Build history of the part. All positions in model axes, mm. A direction names the side the tool comes from. Coordinates: 2 decimals unless noted, no trailing zeros. Order: outer loops, then holes, each group sorted by start corner. A loop starts at its lowest first (then second) coordinate and runs counter-clockwise, first axis right, second up. Notation, with made-up numbers: (10.25, -7) - (16.25, -7) arc R21 ccw to (16.25, 7) - close; hole circle Ø10 at (22, 80). An arc over 180 degrees is marked (long way). Write each question's results on one line, items separated by ' | '. Start each with the question number.
Autodesk Inventor part; units mm, degrees
ref_plane "YZ Plane" through (0, 0, 0) normal (1, 0, 0) x (0, 1, 0)
ref_plane "XZ Plane" through (0, 0, 0) normal (0, 1, 0) x (-1, 0, 0)
ref_plane "XY Plane" through (0, 0, 0) normal (0, 0, 1) x (1, 0, 0)
sketch "スケッチ1" plane through (0, 0, 0) normal (0, 0, 1) x (1, 0, 0)
  line L0 (-47, 28.25) -> (-37.7144, 28.25)
  line L1 (47, 28.25) -> (47, 23.75)
  line L2 (47, -28.25) -> (-47, -28.25)
  line L3 (-47, -28.25) -> (-47, -11.5167)
  line L4 (-47, 28.25) -> (47, -28.25) construction
  line L5 (47, 28.25) -> (-47, -28.25) construction
  line L6 (0, 28.25) -> (0, -28.25) construction
  line L7 (-33, 9.4167) -> (-28, 9.4167) construction
  line L8 (-28, 9.4167) -> (-28, -9.4167) construction
  line L9 (-28, -9.4167) -> (-33, -9.4167) construction
  line L10 (-33, -9.4167) -> (-33, 9.4167) construction
  line L11 (-33, 9.4167) -> (-28, -9.4167) construction
  line L12 (-28, 9.4167) -> (-33, -9.4167) construction
  line L13 (-33.05, 9.4667) -> (-27.95, 9.4667)
  line L14 (-27.95, 9.4667) -> (-27.95, 7.3667) construction
  line L15 (-27.95, -9.4667) -> (-33.05, -9.4667)
  line L16 (-33.05, -9.4667) -> (-33.05, -7.3667) construction
  line L17 (-33.05, 9.4667) -> (-27.95, -9.4667) construction
  line L18 (-27.95, 9.4667) -> (-33.05, -9.4667) construction
  arc A0 (-33.05, 9.4667) -> (-33.05, 7.3667) centre (-33.05, 8.4167) ccw
  line L19 (-30.5, 9.4667) -> (-30.5, -9.4667) construction
  arc A1 (-27.95, 7.3667) -> (-27.95, 9.4667) centre (-27.95, 8.4167) ccw
  line L20 (-33.05, 7.3667) -> (-33.05, 9.4667) construction
  line L21 (-27.95, 7.3667) -> (-27.95, -7.3667)
  line L22 (-33.05, -7.3667) -> (-33.05, 7.3667)
  line L23 (-27.95, -7.3667) -> (-27.95, -9.4667) construction
  line L24 (33, 9.4167) -> (28, 9.4167) construction
  line L25 (28, 9.4167) -> (28, -9.4167) construction
  line L26 (28, -9.4167) -> (33, -9.4167) construction
  line L27 (33, -9.4167) -> (33, 9.4167) construction
  line L28 (33, 9.4167) -> (28, -9.4167) construction
  line L29 (28, 9.4167) -> (33, -9.4167) construction
  line L30 (33.05, 9.4667) -> (27.95, 9.4667)
  line L31 (27.95, 9.4667) -> (27.95, 7.3667) construction
  line L32 (27.95, -9.4667) -> (33.05, -9.4667)
  line L33 (33.05, -9.4667) -> (33.05, -7.3667) construction
  line L34 (33.05, 9.4667) -> (27.95, -9.4667) construction
  line L35 (27.95, 9.4667) -> (33.05, -9.4667) construction
  arc A2 (33.05, 7.3667) -> (33.05, 9.4667) centre (33.05, 8.4167) ccw
  line L36 (30.5, 9.4667) -> (30.5, -9.4667) construction
  arc A3 (27.95, 9.4667) -> (27.95, 7.3667) centre (27.95, 8.4167) ccw
  line L37 (33.05, 7.3667) -> (33.05, 9.4667) construction
  line L38 (27.95, 7.3667) -> (27.95, -7.3667)
  line L39 (33.05, -7.3667) -> (33.05, 7.3667)
  line L40 (27.95, -7.3667) -> (27.95, -9.4667) construction
  line L41 (-52, 9.4167) -> (-52, -9.4167)
  line L42 (-52, 9.4167) -> (-47, 9.4167)
  arc A4 (-47, 9.4167) -> (-47, 11.5167) centre (-47, 10.4667) ccw
  line L43 (-47, 11.5167) -> (-47, 23.75)
  line L44 (-47, -11.5167) -> (-47, 11.5167)
  line L45 (52, 9.4167) -> (52, -9.4167)
  line L46 (52, 9.4167) -> (47, 9.4167)
  arc A5 (47, 11.5167) -> (47, 9.4167) centre (47, 10.4667) ccw
  line L47 (47, 11.5167) -> (47, -11.5167)
  line L48 (47, -11.5167) -> (47, -28.25)
  line L49 (-52, 0) -> (52, 0) construction
  line L50 (-52, -9.4167) -> (-47, -9.4167)
  arc A6 (-47, -11.5167) -> (-47, -9.4167) centre (-47, -10.4667) ccw
  arc A7 (47, -9.4167) -> (47, -11.5167) centre (47, -10.4667) ccw
  line L51 (52, -9.4167) -> (47, -9.4167)
  line L52 (-33.05, 0) -> (-27.95, 0) construction
  arc A8 (-33.05, -7.3667) -> (-33.05, -9.4667) centre (-33.05, -8.4167) ccw
  arc A9 (-27.95, -9.4667) -> (-27.95, -7.3667) centre (-27.95, -8.4167) ccw
  arc A10 (27.95, -7.3667) -> (27.95, -9.4667) centre (27.95, -8.4167) ccw
  arc A11 (33.05, -9.4667) -> (33.05, -7.3667) centre (33.05, -8.4167) ccw
  arc A12 (-47, 24.0838) -> (-37.7144, 28.25) centre (-44.75, 31.5) ccw
  arc A13 (37.7144, 28.25) -> (47, 24.0838) centre (44.75, 31.5) ccw
  line L53 (-47, 24.0838) -> (-47, 28.25)
  line L54 (-37.7144, 28.25) -> (47, 28.25)
  arc A14 (-37.7144, 28.25) -> (-47, 24.0838) centre (-44.75, 31.5) ccw
  arc A15 (47, 24.0838) -> (37.7144, 28.25) centre (44.75, 31.5) ccw
  line L55 (-44.75, 23.75) -> (-47, 23.75)
  line L56 (44.75, 23.75) -> (47, 23.75)
  line L57 (-47, 23.75) -> (-47, 24.0838)
  line L58 (47, 23.75) -> (47, 11.5167)
  line L59 (-23, 23.25) -> (23, 23.25)
  line L60 (23, 23.25) -> (23, -23.25)
  line L61 (23, -23.25) -> (-23, -23.25)
  line L62 (-23, -23.25) -> (-23, 23.25)
  line L63 (-23, 23.25) -> (23, -23.25) construction
  line L64 (23, 23.25) -> (-23, -23.25) construction
  line L65 (-42, 8.25) -> (42, 8.25) construction
  line L66 (42, 8.25) -> (42, -18.25) construction
  line L67 (42, -18.25) -> (-42, -18.25) construction
  line L68 (-42, -18.25) -> (-42, 8.25) construction
  line L69 (-42, 8.25) -> (42, -18.25) construction
  line L70 (42, 8.25) -> (-42, -18.25) construction
  circle A16 centre (-39, 5.25) radius 1.25
  line L71 (-42, -5) -> (42, -5) construction
  circle A17 centre (-39, -15.25) radius 1.25
  circle A18 centre (39, 5.25) radius 1.25
  circle A19 centre (39, -15.25) radius 1.25
  point P0 (0, 0)
  point P1 (-30.5, 0)
  point P2 (30.5, 0)
  point P3 (0, 0)
  point P4 (-30.5, 0)
  point P5 (-30.5, 0)
  point P6 (0, 0)
  point P7 (0, 0)
  point P8 (47, 9.4167)
  point P9 (47, 9.4167)
  point P10 (0, -5)
  point P11 (0, -5)
  dimension "d0" = 94
  dimension "d1" = 56.5
  dimension "d2" = 5
  dimension "d3" = 18.8333
  dimension "d4" = 1.05
  dimension "d5" = 0.05
  dimension "d6" = 0.05
  dimension "d7" = 56
  dimension "d10" = 1.05
  dimension "d11" = 5
  dimension "d34" = 18.8333
  dimension "d40" = 31.5
  dimension "d41" = 89.5
  dimension "d42" = 15.5
  dimension "d43" = 52
  dimension "d60" = 5
  dimension "d63" = 5
  dimension "d69" = 5
  dimension "d70" = 20
  dimension "d71" = 10
  dimension "d72" = 84
  dimension "d73" = 26.5
  dimension "d78" = 2.5
  dimension "d80" = 3
  dimension "d81" = 3
extrude "押し出し1" add sketch "スケッチ1" along normal blind 5 contours L54 A13 L56 L58 A5 L47 A7 L48 L2 L3 A6 L44 A4 L43 L55 A12
extrude "押し出し2" add sketch "スケッチ1" along normal blind 2.5 contours L44 L50 L41 L42 | L46 L45 L51 L47
sketch "スケッチ2" plane through (47, 11.5167, 0) normal (1, 0, 0) x (0, 0, -1)
  line L0 (0, -23.0333) -> (-5, -23.0333)
  line L1 (-2.5, -23.0333) -> (-2.5, -39.7667)
  line L2 (0, -39.7667) -> (-5, -39.7667)
  line L3 (0, -2.1) -> (-2.5, -2.1)
  line L4 (0, -20.9333) -> (-2.5, -20.9333)
  point P0 (0, -11.5167)
  point P1 (-2.5, 7.9)
  dimension "d67" = 10
hole "穴1" at (47, 19.4167, 2.5) direction (-1, 0, 0) diameter 2.459 depth 10 tip angle 118
sketch "スケッチ3" plane through (-47, 11.5167, 0) normal (-1, 0, 0) x (0, 0, 1)
  circle A0 centre (2.5, 7.9) radius 1.2295
  circle A1 centre (2.5, -30.9333) radius 1.2295
  point P0 (0, -11.5167)
  point P1 (2.5, 7.9)
hole "穴2" at (-47, 19.4167, 2.5) direction (1, 0, 0) diameter 2.459 depth 10 tip angle 118
fillet "フィレット1" radius 1 4 edges at (-23, 23.25, 2.5) (-23, -23.25, 2.5) (23, -23.25, 2.5) (23, 23.25, 2.5)
equation "\"d3\" = d34"
equation "\"d6\" = d5"
equation "\"d10\" = d4"
properties part number "Cockpit_horizontal_frame_04" material "アセタール樹脂、黒"
Item 1: Slice it at A-A (y = 1). Write the cut outline in (x, z), then the cut area to 3 significant figures.
Item 2: Probe probe 1 along X at (y, z) = (-3, 3.3); probe 2 along Y at (x, z) = (-5, 3.6); probe 3 along X at (y, z) = (16, 4.2). List the from-to ranges inside material, lowest first.
Item 3: Slice it at C-C (y = -19.5). Write the cut outline in (x, z).
Item 4: Slice it at B-B (x = -9). Write the cut outline in (y, z).
Item 5: Flat gauge pins, fed straight in: P1, Ø1.5, axis at x = -48.5, y = -3, coming from the +Z side; P2, Ø4, axis at x = 20, y = 4, coming from the -Z side; P3, Ø0.8, axis at x = 50, z = 2, coming from the +Y side; P4, Ø2, axis at y = -21, z = 2.5, coming from the +X side. Where does each tip first touch, or does it go through?
Item 6: Which spindle directions (+Z, -Z, +X, -X, +Y, -Y) get a long thin tool onto all of the face, cutting with end or side? Do faces 1 (the flat face through (49, 0, 2.5)), 2 (the flat face through (47, -20, 2)), 3 (the flat face through (-50, 9.417, 1)), 4 (the flat face through (0, 23.25, 2)), 5 (the flat face through (-47, 0, 4)). Say none if no direction does.
Item 7: Pull direction X, two halves, no side cores. Call faces 6 (the cylindrical face through (38, 6, 2)), 7 (the cylindrical face through (41.93, 18.198, 2.66)), 8 (the flat face through (-47, 18, 2)): released by +X, released by -X, zero draft, split by the parting line, or undercut.
Resolved:
1) outline: (-52, 0) - (-33.05, 0) - (-33.05, 5) - (-47, 5) - (-47, 2.5) - (-52, 2.5) - close; (-27.95, 0) - (-23, 0) - (-23, 5) - (-27.95, 5) - close; (23, 0) - (27.95, 0) - (27.95, 5) - (23, 5) - close; (33.05, 0) - (52, 0) - (52, 2.5) - (47, 2.5) - (47, 5) - (33.05, 5) - close | area: 214 mm^2
2) probe 1: -47 to -33.05, -27.95 to -23, 23 to 27.95, 33.05 to 47 | probe 2: -28.25 to -23.25, 23.25 to 28.25 | probe 3: -47 to -23, 23 to 47
3) outline: (-47, 0) - (-23, 0) - (-23, 5) - (-47, 5) - close; (23, 0) - (47, 0) - (47, 5) - (23, 5) - close
4) outline: (-28.25, 0) - (-23.25, 0) - (-23.25, 5) - (-28.25, 5) - close; (23.25, 0) - (28.25, 0) - (28.25, 5) - (23.25, 5) - close
5) P1: z = 2.5 | P2: through | P3: y = 9.42 | P4: x = 47
6) face 1: +Z, +X, +Y, -Y | face 2: +Z, -Z, +X, -Y | face 3: +Z, -Z, -X, +Y | face 4: +Z, -Z | face 5: +Z, -X, +Y, -Y
7) face 6: undercut | face 7: zero draft | face 8: released by -X
